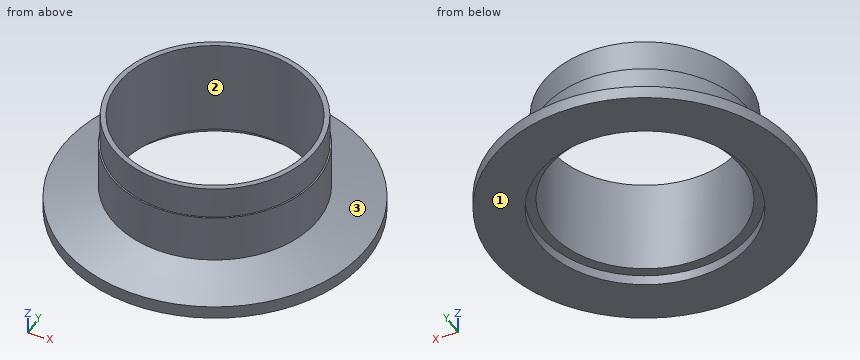
```python
from build123d import *

# Parameters (mm, degrees)
SKETCH2_W = 21.629907471
SKETCH2_H = 12.119969406


with BuildPart() as part:
    # Sketch1 → Revolve1 (revolve)
    with BuildSketch(Plane(origin=(0, 0, 0), x_dir=(0, 0, -1), z_dir=(1, 0, 0)), mode=Mode.PRIVATE) as revolve1_sk:
        Polygon((0, 26.1112), (-2.54, 26.1112), (-2.54, 23.749), (-26.2128, 23.749), (-26.2128, 25.4), (-6.407807007, 25.4), (-3.175, 37.465), (0, 37.465), align=None)
    revolve(revolve1_sk.sketch.rotate(Axis((0, 0, 56.040860285), (0, 0, -1)), 90), axis=Axis((0, 0, 56.040860285), (0, 0, -1)))

    # Sketch2 → Cut-Revolve1 (revolve, cut)
    with BuildSketch(Plane(origin=(0, 0, 0), x_dir=(0, 0, -1), z_dir=(1, 0, 0)), mode=Mode.PRIVATE) as cut_revolve1_sk:
        with Locations((-29.077553736, 31.078984703)):
            Rectangle(SKETCH2_W, SKETCH2_H)
    revolve(cut_revolve1_sk.sketch.rotate(Axis((0, 0, 38.126599349), (0, 0, 1)), 270), axis=Axis((0, 0, 38.126599349), (0, 0, 1)), mode=Mode.SUBTRACT)


solid = part.part
```
Work out the finished part from the listing and answer in its coordinate system (mm). Face numbers are marked on the shaded views. Give positions to 0.01 mm unless a question says otherwise; leave off trailing zeros. Write each loop counter-clockwise with the first axis right and the second up, starting at its lowest first coordinate (ties: lowest second). Pieces come first, ordered by that corner, then holes.
(1) Straight lines are drawn through the part: line 1 (Y direction, x = 0, z = 1.5) (3 decimals); line 2 (X direction, y = 0.5, z = 17.75); line 3 (Y direction, x = 11, z = 25). For each, find the intervals that lie inside material, in ascending order.
Final values:
line 1: y = -37.465 to -26.111, 26.111 to 37.465
line 2: x = -25.4 to -23.74, 23.74 to 25.4
line 3: y = -22.47 to -21.05, 21.05 to 22.47
(2) Flat-ended cylindrical pins translate along their axes: pin 1 Ø3 at (x, y) = (21, 3.5) entering from -Z; pin 2 Ø6 at (y, z) = (0.5, 12) entering from -X; pin 3 Ø5 at (x, z) = (-14, 19.5) entering from +Y; pin 4 Ø8 at (y, z) = (-28.5, 4.5) entering from -X. Find the tip coordinate at first contact, or state that the pin passes through.
Final values:
pin 1: passes through
pin 2: stops at x = -25.4
pin 3: stops at y = 22.48
pin 4: stops at x = -28.15
(3) The part is cut by section C-C on z = 21. Write down the section's boundary in (x, y).
Final values:
outline: circle Ø50.04 at (0, 0); hole circle Ø47.5 at (0, 0)
(4) The mould has two halves that part along X. Classify the marked faces 1, 2 and 3: pulls with the +X half, pulls with the -X half, needs draft (parallel to the pull), parting line crosses it, or undercut.
Final values:
face 1: needs draft
face 2: undercut
face 3: parting line crosses it
(5) The part is cut by section A-A on x = 0. Write down the section's boundary in (y, z) (3 decimals), plus the area to 3 significant figures.
Final values:
outline: (-37.465, 0) - (-26.111, 0) - (-26.111, 2.54) - (-23.749, 2.54) - (-23.749, 26.213) - (-25.019, 26.213) - (-25.019, 18.263) - (-25.4, 18.263) - (-25.4, 6.408) - (-37.465, 3.175) - close; (23.749, 2.54) - (26.111, 2.54) - (26.111, 0) - (37.465, 0) - (37.465, 3.175) - (25.4, 6.408) - (25.4, 18.263) - (25.019, 18.263) - (25.019, 26.213) - (23.749, 26.213) - close
area: 184 mm2
